Check sheet for the drawn part. Datum: minimum x, y, z corner. Units: mm. A direction names the side the tool comes from. Round coordinates to 2 decimals unless told otherwise and drop trailing zeros. Write each loop counter-clockwise with the first axis right and the second up, starting at its lowest first coordinate (ties: lowest second). Pieces come first, ordered by that corner, then holes. Notation, with made-up numbers: (-29.75, -6.75) - (6.25, -6.75) arc R30 cw to (6.25, 27.25) - close; hole circle Ø5 at (74.25, -38.75). An arc over 180 degrees is marked (long way). Write each question's results on one line, items separated by ' | '.
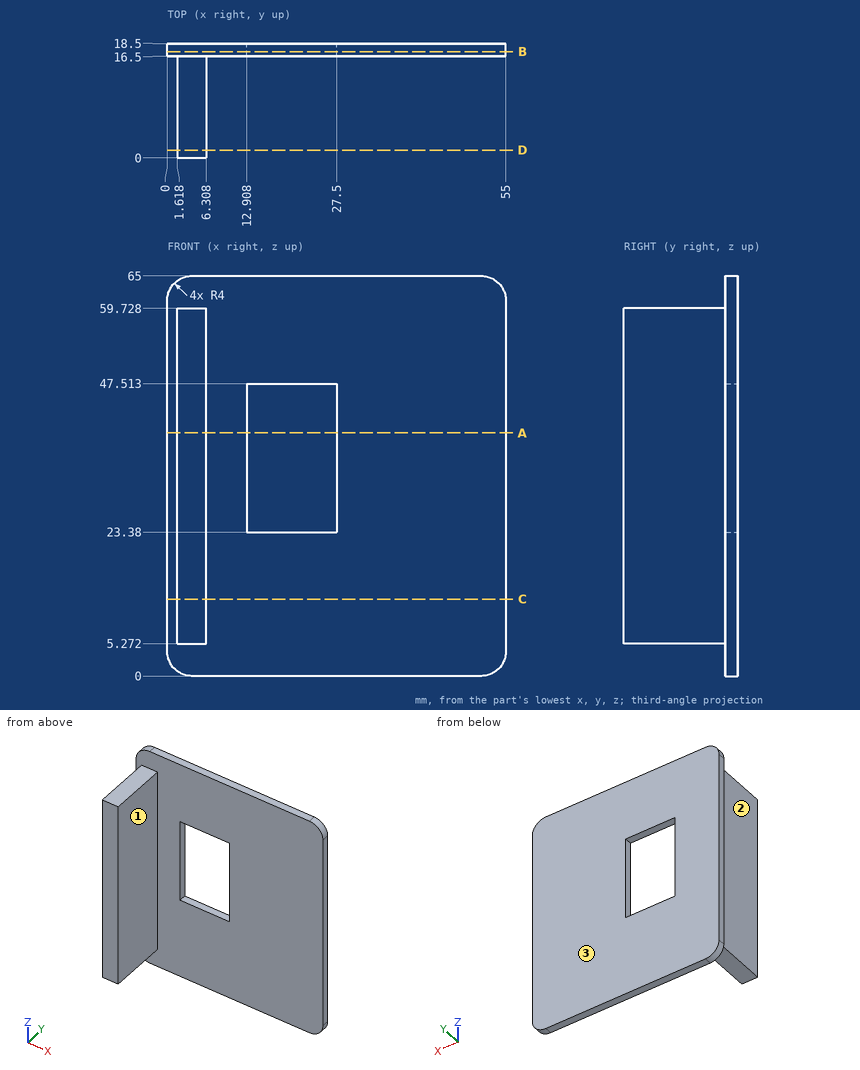
(1) Section check C-C (z = 12.5). Record the cut outline in (x, y).
Answer:
outline: (0, 16.5) - (1.62, 16.5) - (1.62, 0) - (6.31, 0) - (6.31, 16.5) - (55, 16.5) - (55, 18.5) - (0, 18.5) - close
(2) Thickness scan on L1, parallel to Z at x = 19.5, y = 17.5; L2, parallel to X at y = 1.5, z = 48; L3, parallel to Z at x = 3, y = 14.5. Record the ranges inside material, lowest first.
Answer:
L1: 0 to 23.38, 47.51 to 65 | L2: 1.62 to 6.31 | L3: 5.27 to 59.73
(3) Go/stop test with flat-tipped pins: pin 1 Ø5 at (x, y) = (4.5, 10.5) entering from -Z; pin 2 Ø12 at (x, z) = (19, 46) entering from -Y; pin 3 Ø8 at (y, z) = (7.5, 30) entering from -X; pin 4 Ø2 at (x, y) = (24, 17.5) entering from -Z. Record where each tip stops, or that it passes through.
Answer:
pin 1: z = 5.27 | pin 2: y = 16.5 | pin 3: x = 1.62 | pin 4: z = 0
(4) Set-up check for the marked faces 1, 2 and 3: record each of +Z, -Z, +X, -X, +Y, -Y from which the full face is reachable in a straight line by a thin tool's end or side.
Answer:
face 1: +Z, -Z, +X, -Y | face 2: +Z, -Z, -X, -Y | face 3: +Z, -Z, +X, -X, +Y
(5) Section check B-B (y = 17.25). Record the cut outline in (x, z), plus the area to 3 significant figures.
Answer:
outline: (0, 4) arc R4 ccw to (4, 0) - (51, 0) arc R4 ccw to (55, 4) - (55, 61) arc R4 ccw to (51, 65) - (4, 65) arc R4 ccw to (0, 61) - close; hole (12.91, 23.38) - (27.5, 23.38) - (27.5, 47.51) - (12.91, 47.51) - close | area: 3,210 mm2
(6) Section check A-A (z = 39.5). Record the cut outline in (x, y).
Answer:
outline: (0, 16.5) - (1.62, 16.5) - (1.62, 0) - (6.31, 0) - (6.31, 16.5) - (12.91, 16.5) - (12.91, 18.5) - (0, 18.5) - close; (27.5, 16.5) - (55, 16.5) - (55, 18.5) - (27.5, 18.5) - close
(7) Section check D-D (y = 1.25). Record the cut outline in (x, z), plus the area to 3 significant figures.
Answer:
outline: (1.62, 5.27) - (6.31, 5.27) - (6.31, 59.73) - (1.62, 59.73) - close | area: 255 mm2
